```python
from build123d import *

# Parameters (mm, degrees)
SKETCH1_W          = 83.82
SKETCH1_H          = 25.4
BOX_DEPTH          = 6.35
CUT_EXTRUDE1_DEPTH = 3.175


with BuildPart() as part:
    # Sketch1 → Box (new body)
    with BuildSketch(Plane(origin=(0, 0, 0), x_dir=(1, 0, 0), z_dir=(0, 1, 0))):
        Rectangle(SKETCH1_W, SKETCH1_H)
    extrude(amount=BOX_DEPTH)

    # Sketch5 → Cut-Extrude1 (cut)
    with BuildSketch(Plane(origin=(0, 0, 0), x_dir=(1, 0, 0), z_dir=(0, 1, 0))):
        with BuildLine():
            Line((-13.354872806, -5.08), (-20.935127194, -5.08))
            ThreePointArc((-20.935127194, -5.08), (-26.015127194, 0), (-20.935127194, 5.08))
            Line((-20.935127194, 5.08), (-13.354872806, 5.08))
            ThreePointArc((-13.354872806, 5.08), (-8.274872806, 0), (-13.354872806, -5.08))
        make_face()
        with BuildLine():
            Line((13.354872806, -5.08), (20.935127194, -5.08))
            ThreePointArc((20.935127194, -5.08), (26.015127194, 0), (20.935127194, 5.08))
            Line((20.935127194, 5.08), (13.354872806, 5.08))
            ThreePointArc((13.354872806, 5.08), (8.274872806, 0), (13.354872806, -5.08))
        make_face()
    extrude(amount=CUT_EXTRUDE1_DEPTH, mode=Mode.SUBTRACT)


solid = part.part
```
The model under review builds one solid part; all positions refer to its coordinate system, in mm. A direction names the side the tool comes from. Round coordinates to 2 decimals unless told otherwise and drop trailing zeros. Loops run counter-clockwise (first coordinate to the right, second up) from the corner with the lowest first, then second, coordinate; pieces in that order, holes last. Notation, with made-up numbers: M 9.25,45.5 L 36.25,45.5 A27 ccw 36.25,62.5 Z; hole C -12,-14 d5. An arc over 180 degrees is marked long. Answer as a JSON object with one key per item and string values.
(1) Take a section at B-B on x = -15. Give the boundary of the cut face in (y, z) (3 decimals), and give its area (3 significant figures).
Resolved:
{"outline": "M 0,-12.7 L 6.35,-12.7 L 6.35,12.7 L 0,12.7 L 0,5.08 L 3.175,5.08 L 3.175,-5.08 L 0,-5.08 Z", "area": "129 mm²"}
(2) Tool access review of faces 5 (the flat face through (-1, 0, 0)), 6 (the flat face through (-17, 2, 5.08)): name each direction out of +Z, -Z, +X, -X, +Y, -Y from which nothing blocks a thin tool from reaching the whole face with its end or side.
Resolved:
{"face 5": "+Z, -Z, +X, -X, -Y", "face 6": "-Y"}
(3) Draft analysis for pull direction Z (two halves, no side actions). For faces 1 (the cylindrical face through (-26.014, 1.565, 0.112)), 2 (the flat face through (-1, 3, -12.7)), 3 (the flat face through (41.91, 3, 0)), 4 (the flat face through (17, 2, -5.08)), state which applies: released by +Z, released by -Z, zero draft, split by the parting line, or undercut.
Resolved:
{"face 1": "undercut", "face 2": "released by -Z", "face 3": "zero draft", "face 4": "undercut"}
(4) Clearance check with flat-ended pins moving along their axes: P1, Ø8, axis at x = 13, z = 1.5, coming from the -Y side; P2, Ø3, axis at x = -12.5, z = 0.5, coming from the -Y side (3 decimals). State where each tip first meets the part, or that it passes through.
Resolved:
{"P1": "y = 0", "P2": "y = 3.175"}
(5) To check wall thickness, follow line 1 along X through (y, z) = (3, 1); line 2 along Z through (x, y) = (-23.5, 2.5). State the ranges of each line that lie inside material, in increasing order.
Resolved:
{"line 1": "-41.91 to -25.92, -8.37 to 8.37, 25.92 to 41.91", "line 2": "-12.7 to -4.38, 4.38 to 12.7"}
(6) Take a section at A-A on z = 0. Give the boundary of the cut face in (x, y) (3 decimals).
Resolved:
{"outline": "M -41.91,0 L -26.015,0 L -26.015,3.175 L -8.275,3.175 L -8.275,0 L 8.275,0 L 8.275,3.175 L 26.015,3.175 L 26.015,0 L 41.91,0 L 41.91,6.35 L -41.91,6.35 Z"}
(7) Take a section at C-C on x = 22. Give the boundary of the cut face in (y, z) (3 decimals), and give its area (3 significant figures).
Resolved:
{"outline": "M 0,-12.7 L 6.35,-12.7 L 6.35,12.7 L 0,12.7 L 0,4.967 L 3.175,4.967 L 3.175,-4.967 L 0,-4.967 Z", "area": "130 mm²"}
